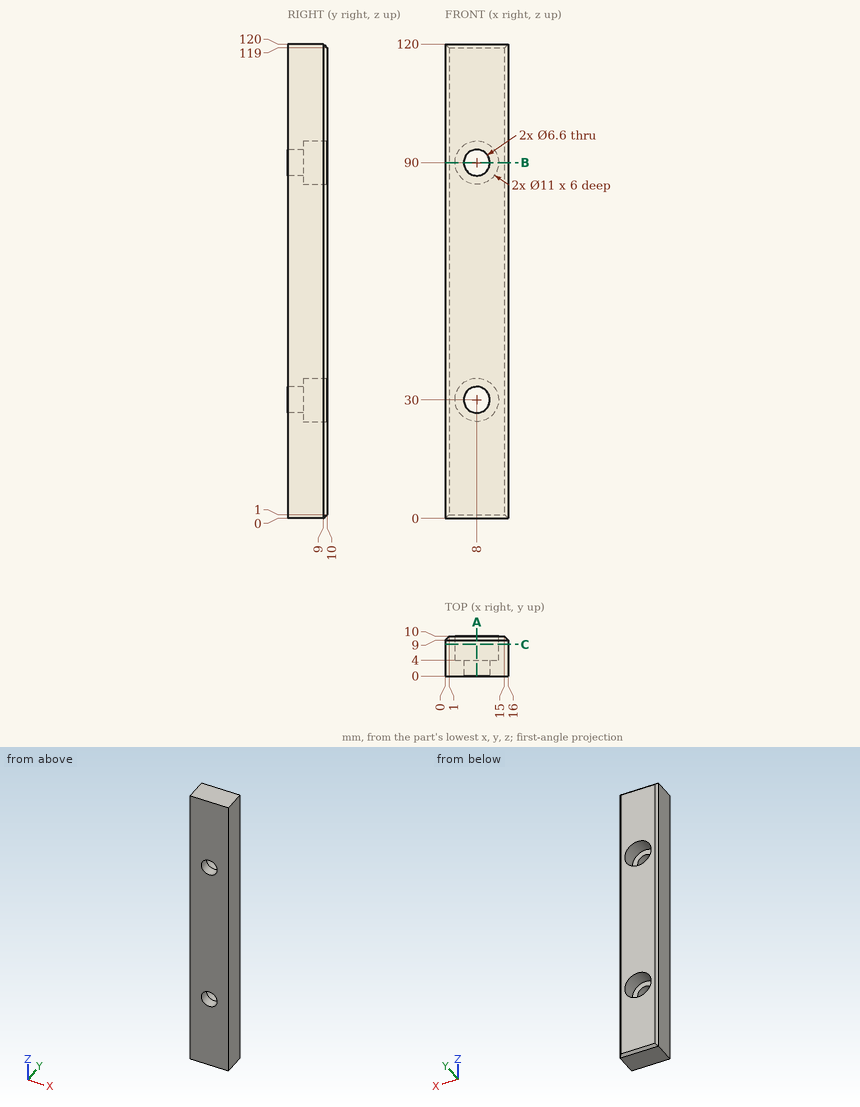
Verification items for this drawing (mm, ordinates from the low corner). Coordinates: 2 decimals unless noted, no trailing zeros. Write each loop counter-clockwise with the first axis right and the second up, starting at its lowest first coordinate (ties: lowest second). Pieces come first, ordered by that corner, then holes. Notation, with made-up numbers: (35, 51) -> (83, 51) arc R11 ccw to (83, 69) -> close; hole circle Ø4 at (-37.5, -12.5). An arc over 180 degrees is marked (long way). One line per item, written item: value. Start each with the question number.
Q1. Thickness scan on L1, parallel to Z at x = 8, y = 2; L2, parallel to Z at x = 8, y = 6.05. Record the ranges inside material, lowest first. Write a range as from..to.
Q2. Cross-section at C-C on y = 8. Enter the section's corners in (x, z), and give its area (3 significant figures).
Q3. Cross-section at B-B on z = 90. Enter the section's corners in (x, y).
Q4. Cross-section at A-A on x = 8. Enter the section's corners in (y, z), and give its area (3 significant figures).
Q5. Go/stop test with a flat-tipped pin: P1, Ø6, axis at x = 8, z = 30, coming from the -Y side. Record where the tip stops, or that it passes through.
Checked values:
1. L1: z = 0..26.7, 33.3..86.7, 93.3..120
1. L2: z = 0..24.5, 35.5..84.5, 95.5..120
2. outline: (0, 0) -> (16, 0) -> (16, 120) -> (0, 120) -> close; hole circle Ø11 at (8, 30); hole circle Ø11 at (8, 90)
2. area: 1,730 mm²
3. outline: (0, 0) -> (4.7, 0) -> (4.7, 4) -> (2.5, 4) -> (2.5, 10) -> (1, 10) -> (0, 9) -> close; (11.3, 0) -> (16, 0) -> (16, 9) -> (15, 10) -> (13.5, 10) -> (13.5, 4) -> (11.3, 4) -> close
4. outline: (0, 0) -> (9, 0) -> (10, 1) -> (10, 24.5) -> (4, 24.5) -> (4, 26.7) -> (0, 26.7) -> close; (0, 33.3) -> (4, 33.3) -> (4, 35.5) -> (10, 35.5) -> (10, 84.5) -> (4, 84.5) -> (4, 86.7) -> (0, 86.7) -> close; (0, 93.3) -> (4, 93.3) -> (4, 95.5) -> (10, 95.5) -> (10, 119) -> (9, 120) -> (0, 120) -> close
4. area: 1,010 mm²
5. P1: passes through
